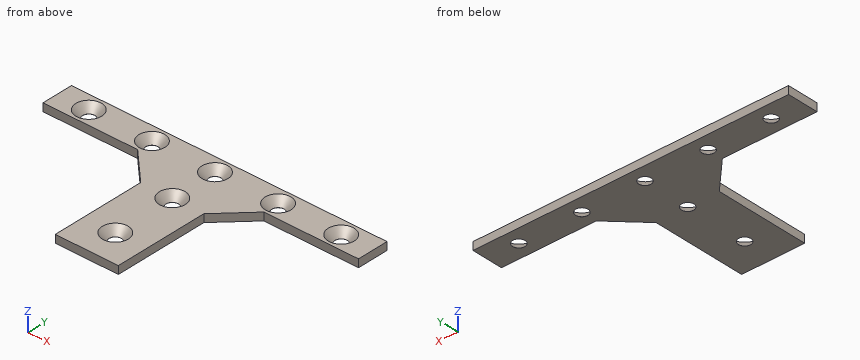
```python
from build123d import *

# Parameters (mm, degrees)
BOSS_EXTRUDE1_DEPTH             = 3.175
F_10_CLEARANCE_HOLE1_AT_2_COUNT = 2
F_10_CLEARANCE_HOLE1_AT_2_PITCH = 25.4
F_10_CLEARANCE_HOLE1_AT_3_COUNT = 2
F_10_CLEARANCE_HOLE1_AT_3_PITCH = 50.8
F_10_CLEARANCE_HOLE1_AT_4_COUNT = 2
F_10_CLEARANCE_HOLE1_AT_4_PITCH = 101.6
F_10_CLEARANCE_HOLE1_AT_5_COUNT = 2
F_10_CLEARANCE_HOLE1_AT_5_PITCH = 54.254423783
F_10_CLEARANCE_HOLE1_AT_6_COUNT = 2
F_10_CLEARANCE_HOLE1_AT_6_PITCH = 67.501425911
F_10_CLEARANCE_HOLE1_AT_7_COUNT = 2
F_10_CLEARANCE_HOLE1_AT_7_PITCH = 76.2


with BuildPart() as part:
    # Sketch1 → Boss-Extrude1 (new body)
    with BuildSketch(Plane.XY):
        Polygon((41.275, -25.4), (41.275, -63.5), (66.675, -63.5), (66.675, -25.4), (79.375, -12.7), (117.475, -12.7), (117.475, 0), (-9.525, 0), (-9.525, -12.7), (28.575, -12.7), align=None)
    extrude(amount=BOSS_EXTRUDE1_DEPTH)

    # Sketch5 → #10 Clearance Hole1 (revolve, cut)
    with BuildSketch(Plane(origin=(3.175, -6.35, 3.175), x_dir=(0, -1, 0), z_dir=(1, 0, 0))):
        Polygon((0, 0), (0, 3.175), (2.4892, 3.175), (2.4892, 3.141080936), (5.2197, 0), align=None)
    f_10_clearance_hole1 = revolve(axis=Axis((3.175, -6.35, 9.525), (0, 0, -1)), mode=Mode.SUBTRACT)

    # #10 Clearance Hole1 at 2: #10 Clearance Hole1 ×2
    with Locations(*[(i * F_10_CLEARANCE_HOLE1_AT_2_PITCH, 0, 0) for i in range(1, F_10_CLEARANCE_HOLE1_AT_2_COUNT)]):
        add(f_10_clearance_hole1, mode=Mode.SUBTRACT)

    # #10 Clearance Hole1 at 3: #10 Clearance Hole1 ×2
    with Locations(*[(i * F_10_CLEARANCE_HOLE1_AT_3_PITCH, 0, 0) for i in range(1, F_10_CLEARANCE_HOLE1_AT_3_COUNT)]):
        add(f_10_clearance_hole1, mode=Mode.SUBTRACT)

    # #10 Clearance Hole1 at 4: #10 Clearance Hole1 ×2
    with Locations(*[(i * F_10_CLEARANCE_HOLE1_AT_4_PITCH, 0, 0) for i in range(1, F_10_CLEARANCE_HOLE1_AT_4_COUNT)]):
        add(f_10_clearance_hole1, mode=Mode.SUBTRACT)

    # #10 Clearance Hole1 at 5: #10 Clearance Hole1 ×2
    with Locations(*[Vector(0.9363291775690471, -0.35112344158838477, 0) * (i * F_10_CLEARANCE_HOLE1_AT_5_PITCH) for i in range(1, F_10_CLEARANCE_HOLE1_AT_5_COUNT)]):
        add(f_10_clearance_hole1, mode=Mode.SUBTRACT)

    # #10 Clearance Hole1 at 6: #10 Clearance Hole1 ×2
    with Locations(*[Vector(0.7525766947068834, -0.6585046078685118, 0) * (i * F_10_CLEARANCE_HOLE1_AT_6_PITCH) for i in range(1, F_10_CLEARANCE_HOLE1_AT_6_COUNT)]):
        add(f_10_clearance_hole1, mode=Mode.SUBTRACT)

    # #10 Clearance Hole1 at 7: #10 Clearance Hole1 ×2
    with Locations(*[(i * F_10_CLEARANCE_HOLE1_AT_7_PITCH, 0, 0) for i in range(1, F_10_CLEARANCE_HOLE1_AT_7_COUNT)]):
        add(f_10_clearance_hole1, mode=Mode.SUBTRACT)


solid = part.part
```
Could you check a few things on this model? Use its own coordinates, in mm. Coordinates: 2 decimals unless noted, no trailing zeros. Write each loop counter-clockwise with the first axis right and the second up, starting at its lowest first coordinate (ties: lowest second). Pieces come first, ordered by that corner, then holes. Notation, with made-up numbers: (69.25, 63.5) -> (80.25, 63.5) arc R28 cw to (80.25, 99.5) -> close; hole circle Ø2 at (22.25, -10). An arc over 180 degrees is marked (long way). Return JSON: item names as keys, results as strings.
(1) Imagine slicing it at A-A, the plane y = -50.8. Please give me the cut outline in (x, z) (3 decimals), then the cut area to 3 significant figures.
Numbers:
{"outline": "(41.275, 0) -> (51.486, 0) -> (51.486, 0.034) -> (48.755, 3.175) -> (41.275, 3.175) -> close; (56.464, 0) -> (66.675, 0) -> (66.675, 3.175) -> (59.195, 3.175) -> (56.464, 0.034) -> close", "area": "56.3 mm2"}
(2) I need wall thicknesses on L1, parallel to Y at x = 57, z = 1.45; L2, parallel to X at y = -44.5, z = 1.1 (3 decimals); L3, parallel to Y at x = 112, z = 2.8. Which ranges of each line are inside material? Lowest first, please.
Numbers:
{"L1": "y = -63.5 to -52.97, -48.63 to -27.57, -23.23 to -8.52, -4.18 to 0", "L2": "x = 41.275 to 66.675", "L3": "y = -12.7 to 0"}
(3) Imagine slicing it at D-D, the plane y = -17. Please give me the cut outline in (x, z) (3 decimals).
Numbers:
{"outline": "(32.875, 0) -> (75.075, 0) -> (75.075, 3.175) -> (32.875, 3.175) -> close"}
(4) Imagine slicing it at B-B, the plane y = -6.35. Count the separate pieces of the cut face and the enclosed holes in it, then the cut area to 3 significant figures.
Numbers:
{"separate pieces": "6", "enclosed holes": "0", "area": "281 mm2"}
(5) I'm going to push flat-ended pins straight in: pin 1 (1.5 mm diameter, centred on x = 88.5, z = 0.5, fed in from -Y); pin 2 (1 mm diameter, centred on y = -39.5, z = 1, fed in from +X) (3 decimals); pin 3 (1.5 mm diameter, centred on y = -23.5, z = 2, fed in from +X) (3 decimals). Where does each tip first touch, or does it pass through?
Numbers:
{"pin 1": "stops at y = -12.7", "pin 2": "stops at x = 66.675", "pin 3": "stops at x = 69.325"}
(6) Imagine slicing it at C-C, the plane z = 2.5. Please give me the cut outline in (x, y) (3 decimals), then the cut area to 3 significant figures.
Numbers:
{"outline": "(-9.525, -12.7) -> (28.575, -12.7) -> (41.275, -25.4) -> (41.275, -63.5) -> (66.675, -63.5) -> (66.675, -25.4) -> (79.375, -12.7) -> (117.475, -12.7) -> (117.475, 0) -> (-9.525, 0) -> close; hole circle Ø9.266 at (3.175, -6.35); hole circle Ø9.266 at (28.575, -6.35); hole circle Ø9.266 at (53.975, -50.8); hole circle Ø9.266 at (53.975, -25.4); hole circle Ø9.266 at (53.975, -6.35); hole circle Ø9.266 at (79.375, -6.35); hole circle Ø9.266 at (104.775, -6.35)", "area": "2,590 mm2"}
